Geometry: see drawing. Coordinates: mm, zero at the bounding-box minimum. A direction names the side the tool comes from. Round coordinates to 2 decimals unless told otherwise and drop trailing zeros. Order: outer loops, then holes, each group sorted by start corner. A loop starts at its lowest first (then second) coordinate and runs counter-clockwise, first axis right, second up.
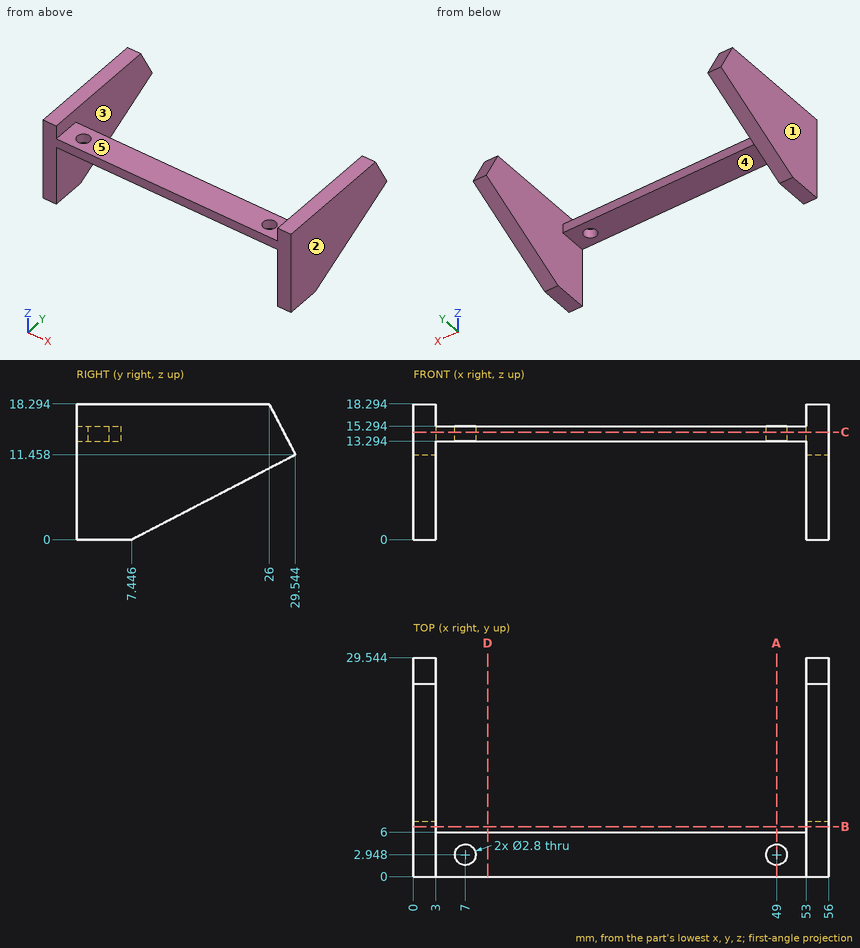
1. Line query: line 1 along X through (y, z) = (17, 14.25); line 2 along Y through (x, z) = (49, 14.5); line 3 along Z through (x, y) = (14, 1.75). Output: solid intervals per line, ascending.
2. First-contact query: pin 1 (1.8 mm diameter, centred on x = 23, y = 2.5, fed in from -Z); pin 2 (12 mm diameter, centred on x = 25, y = 3.5, fed in from +Z); pin 3 (1 mm diameter, centred on x = 16.5, z = 14.5, fed in from +Y); pin 4 (6 mm diameter, centred on y = 13.5, z = 3, fed in from +X). Flat tips, straight axial feed; report the tip coordinate or a pass-through.
3. Section A-A on x = 49. Return loops of the section in (y, z).
4. Access query for the marked faces 4 and 5. Directions: +Z, -Z, +X, -X, +Y, -Y. A direction counts if a zero-diameter tool reaches every point of the face in a straight line with its end or side. Return the directions, or none.
5. Pull-direction query (X, two-part tool) for the marked faces 1, 2 and 3; classes: released by +X, released by -X, zero draft, split by the parting line, or undercut.
6. Section B-B on y = 6.75. Return loops of the section in (x, z).
7. Section D-D on x = 10. Return loops of the section in (y, z).
8. Section C-C on z = 14.5. Return loops of the section in (x, y).
Result:
1. line 1: x = 0 to 3, 53 to 56
1. line 2: y = 0 to 1.55, 4.35 to 6
1. line 3: z = 13.29 to 15.29
2. pin 1: stops at z = 13.29
2. pin 2: stops at z = 15.29
2. pin 3: stops at y = 6
2. pin 4: stops at x = 56
3. outline: (0, 13.29) - (1.55, 13.29) - (1.55, 15.29) - (0, 15.29) - close; (4.35, 13.29) - (6, 13.29) - (6, 15.29) - (4.35, 15.29) - close
4. face 4: -Z, +Y, -Y
4. face 5: +Z, +Y, -Y
5. face 1: released by -X
5. face 2: released by +X
5. face 3: undercut
6. outline: (0, 0) - (3, 0) - (3, 18.29) - (0, 18.29) - close; (53, 0) - (56, 0) - (56, 18.29) - (53, 18.29) - close
7. outline: (0, 13.29) - (6, 13.29) - (6, 15.29) - (0, 15.29) - close
8. outline: (0, 0) - (56, 0) - (56, 27.97) - (53, 27.97) - (53, 6) - (3, 6) - (3, 27.97) - (0, 27.97) - close; hole circle Ø2.8 at (7, 2.95); hole circle Ø2.8 at (49, 2.95)
